Autodesk Fusion 360 part; units mm, degrees
sketch "草图1" plane through (0, 0, 0) normal (0, 0, 1) x (1, 0, 0)
  line L0 (-75, 0) -> (-70, 0) construction
  line L1 (-70, 0) -> (75, 0) construction
  line L2 (0, 50) -> (0, -52.1887) construction
  circle A0 centre (0, 0) radius 7
  circle A1 centre (0, 0) radius 10
  line L3 (-32, 5) -> (-18, 5)
  line L4 (-32, -5) -> (-18, -5)
  line L5 (-32, -3) -> (-18, -3)
  line L6 (-32, 3) -> (-18, 3)
  line L7 (-32, 10) -> (0, 10)
  line L8 (-32, -10) -> (0, -10)
  arc A2 (-32, 5) -> (-32, -5) centre (-32, 0) ccw
  arc A3 (-32, 3) -> (-32, -3) centre (-32, 0) ccw
  arc A4 (-18, -3) -> (-18, 3) centre (-18, 0) ccw
  arc A5 (-18, -5) -> (-18, 5) centre (-18, 0) ccw
  arc A6 (-32, 10) -> (-32, -10) centre (-32, 0) ccw
  dimension "d1" = 5
  dimension "d2" = 14
  dimension "d3" = 3
  dimension "d4" = 5
  dimension "d5" = 3
  dimension "d6" = 20
  dimension "d7" = 14
  dimension "d8" = 18
  dimension "d9" = 14
extrude "拉伸1" add sketch "草图1" along normal blind 8 contours A1 L7 L8 A6
extrude "拉伸2" add sketch "草图1" along normal blind 20 contours A1
extrude "拉伸3" add sketch "草图1" along normal blind 11 contours L3 L4 A2 A5
The listing builds one solid part. Answer for the finished solid, in the listing's coordinates (mm). A direction names the side the tool comes from. Round coordinates to 2 decimals unless told otherwise and drop trailing zeros. Write each loop counter-clockwise with the first axis right and the second up, starting at its lowest first coordinate (ties: lowest second). Pieces come first, ordered by that corner, then holes. Notation, with made-up numbers: (23, 1.25) - (31, 1.25) arc R9 cw to (31, 7.25) - close; hole circle Ø6 at (20.25, 48.5). An arc over 180 degrees is marked (long way). Use a Markdown table: item, result. Add a question column.
1. Flat-ended cylindrical pins translate along their axes: P1, Ø11, axis at x = -25, y = 1, coming from the +Z side; P2, Ø0.9, axis at x = -24.5, z = 9.5, coming from the +Y side; P3, Ø3, axis at y = -3, z = 10.5, coming from the -X side. Find the tip coordinate at first contact, or state that the pin passes through.
2. Consider line 1 (Y direction, x = -19.5, z = 5); line 2 (Y direction, x = 0, z = 14); line 3 (X direction, y = 2.75, z = 3.25). Determine where each line is inside the solid, lowest interval first.
3. For a pull along Y with two mould halves and no side action, classify faces 4 (the face through (-42, 0, 4)), 5 (the face through (-15, 0, 5)), 6 (the face through (-16, -4, 0)) as +Y half, -Y half, draft (parallel to the pull), parting line (faces both ways), or undercut.
4. The part is cut by section C-C (z = 5.5). Write down the section's boundary in (x, y), and give its area (3 significant figures).
5. The part is cut by section B-B (x = -30). Write down the section's boundary in (y, z), and give its area (3 significant figures).
6. The part is cut by section A-A (y = 0). Write down the section's boundary in (x, z).
7. The part is cut by section D-D (z = 18.25). Write down the section's boundary in (x, y).
8. A tool of negligible diameter and unlimited length cuts with its end or side. For faces 1 (the face through (-25, -5, 9)), 2 (the face through (-35, 0, 5)), 3 (the face through (-37, 0, 9)), from which of +Z, -Z, +X, -X, +Y, -Y can it reach the whole face along a straight path? Write none if from no direction.
Reported:
| question | item | result |
|---|---|---|
| 1 | P1 | z = 11 |
| 1 | P2 | y = 5 |
| 1 | P3 | x = -36.77 |
| 2 | line 1 | -10 to -3, 3 to 10 |
| 2 | line 2 | -10 to -7, 7 to 10 |
| 2 | line 3 | -41.61 to -33.2, -16.8 to -6.44, 6.44 to 9.61 |
| 3 | face 4 | parting line |
| 3 | face 5 | undercut |
| 3 | face 6 | draft |
| 4 | outline | (-32, -10) - (0, -10) arc R10 ccw to (0, 10) - (-32, 10) arc R10 ccw to start; hole (-32, -3) - (-18, -3) arc R3 ccw to (-18, 3) - (-32, 3) arc R3 ccw to start; hole circle Ø14 at (0, 0) |
| 4 | area | 688 mm^2 |
| 5 | outline | (-10, 0) - (-3, 0) - (-3, 11) - (-5, 11) - (-5, 8) - (-10, 8) - close; (3, 0) - (10, 0) - (10, 8) - (5, 8) - (5, 11) - (3, 11) - close |
| 5 | area | 124 mm^2 |
| 6 | outline | (-42, 0) - (-35, 0) - (-35, 11) - (-37, 11) - (-37, 8) - (-42, 8) - close; (-15, 0) - (-7, 0) - (-7, 20) - (-10, 20) - (-10, 8) - (-13, 8) - (-13, 11) - (-15, 11) - close; (7, 0) - (10, 0) - (10, 20) - (7, 20) - close |
| 7 | outline | circle Ø20 at (0, 0); hole circle Ø14 at (0, 0) |
| 8 | face 1 | +Z, -X, -Y |
| 8 | face 2 | +Z, -Z |
| 8 | face 3 | +Z, -X |
